from build123d import *

# Parameters (mm, degrees)
SKETCH1_W           = 90
SKETCH1_H           = 30
SKETCH1_R           = 2.5
SKETCH1_R_2         = 4
BOSS_EXTRUDE1_DEPTH = 30
SKETCH4_R           = 2.4
CUT_EXTRUDE1_DEPTH  = 5


with BuildPart() as part:
    # Sketch1 → Boss-Extrude1 (new body)
    with BuildSketch(Plane.XY):
        with Locations((45, 15)):
            Rectangle(SKETCH1_W, SKETCH1_H)
        with Locations((10, 10)):
            Circle(SKETCH1_R, mode=Mode.SUBTRACT)
        with Locations((45, 10)):
            Circle(SKETCH1_R_2, mode=Mode.SUBTRACT)
        with Locations((80, 10)):
            Circle(SKETCH1_R, mode=Mode.SUBTRACT)
    extrude(amount=BOSS_EXTRUDE1_DEPTH)

    # Sketch4 → Cut-Extrude1 (cut)
    with BuildSketch(Plane(origin=(0, 30, 0), x_dir=(1, 0, 0), z_dir=(0, 1, 0))):
        with Locations(Location((7, -8, 0), (0, 0, 270))):
            Circle(SKETCH4_R)
        with Locations(Location((32, -8, 0), (0, 0, 270))):
            Circle(SKETCH4_R)
        with Locations(Location((57, -8, 0), (0, 0, 270))):
            Circle(SKETCH4_R)
        with Locations(Location((82, -8, 0), (0, 0, 270))):
            Circle(SKETCH4_R)
        with Locations(Location((32, -20, 0), (0, 0, 270))):
            Circle(SKETCH4_R)
        with Locations(Location((57, -20, 0), (0, 0, 270))):
            Circle(SKETCH4_R)
        with Locations(Location((82, -20, 0), (0, 0, 270))):
            Circle(SKETCH4_R)
        with Locations(Location((7, -20, 0), (0, 0, 270))):
            Circle(SKETCH4_R)
    extrude(amount=-CUT_EXTRUDE1_DEPTH, mode=Mode.SUBTRACT)


solid = part.part
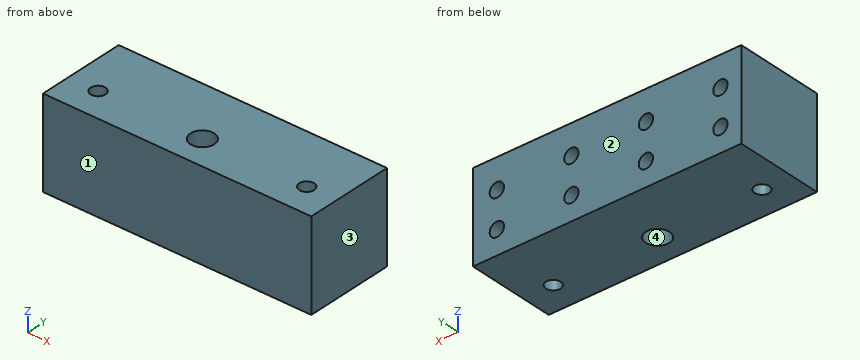
Could you check a few things on this model? Use its own coordinates, in mm. Face numbers are marked on the shaded views. Give positions to 0.01 mm unless a question says otherwise; leave off trailing zeros. Order: outer loops, then holes, each group sorted by start corner. A loop starts at its lowest first (then second) coordinate and runs counter-clockwise, first axis right, second up.
1. Will this pin go through, and if not, where does the flat tip stop? P1, Ø1.4, axis at x = 57, z = 7.5, coming from the +Y side.
2. Suppose I cut it at A-A (x = 45). List the corners of the cut face in (y, z) for me.
3. I need wall thicknesses on L1, parallel to X at y = 27.05, z = 8; L2, parallel to X at y = 26.5, z = 8.75; L3, parallel to Y at x = 10, z = 10.5. Which ranges of each line are inside material? Lowest first, please.
4. Suppose I cut it at C-C (z = 8). List the corners of the cut face in (x, y) for me, plus the area to 3 significant figures.
5. Suppose I cut it at B-B (y = 26.25). Give the number of separate pieces and of enclosed holes in the cut face, plus the area to 3 significant figures.
6. We'd pull the mould along Y, two halves only. Please class the marked faces 1, 2, 3 and 4: pulls with the +Y half, pulls with the -Y half, needs draft (parallel to the pull), parting line crosses it, or undercut.
7. Suppose I cut it at D-D (y = 10). List the corners of the cut face in (x, z) for me.
Solved:
1. P1: stops at y = 25
2. outline: (0, 0) - (6, 0) - (6, 30) - (0, 30) - close; (14, 0) - (30, 0) - (30, 30) - (14, 30) - close
3. L1: x = 0 to 4.6, 9.4 to 29.6, 34.4 to 54.6, 59.4 to 79.6, 84.4 to 90
3. L2: x = 0 to 4.72, 9.28 to 29.72, 34.28 to 54.72, 59.28 to 79.72, 84.28 to 90
3. L3: y = 0 to 7.5, 12.5 to 30
4. outline: (0, 0) - (90, 0) - (90, 30) - (84.4, 30) - (84.4, 25) - (79.6, 25) - (79.6, 30) - (59.4, 30) - (59.4, 25) - (54.6, 25) - (54.6, 30) - (34.4, 30) - (34.4, 25) - (29.6, 25) - (29.6, 30) - (9.4, 30) - (9.4, 25) - (4.6, 25) - (4.6, 30) - (0, 30) - close; hole circle Ø5 at (10, 10); hole circle Ø8 at (45, 10); hole circle Ø5 at (80, 10)
4. area: 2,510 mm2
5. separate pieces: 1
5. enclosed holes: 8
5. area: 2,560 mm2
6. face 1: pulls with the -Y half
6. face 2: pulls with the +Y half
6. face 3: needs draft
6. face 4: undercut
7. outline: (0, 0) - (7.5, 0) - (7.5, 30) - (0, 30) - close; (12.5, 0) - (41, 0) - (41, 30) - (12.5, 30) - close; (49, 0) - (77.5, 0) - (77.5, 30) - (49, 30) - close; (82.5, 0) - (90, 0) - (90, 30) - (82.5, 30) - close
